Autodesk Inventor part; units mm, degrees
ref_plane "YZ Plane" through (0, 0, 0) normal (1, 0, 0) x (0, 1, 0)
ref_plane "XZ Plane" through (0, 0, 0) normal (0, 1, 0) x (-1, 0, 0)
ref_plane "XY Plane" through (0, 0, 0) normal (0, 0, 1) x (1, 0, 0)
sketch "Náčrt1" plane through (0, 0, 0) normal (0, 1, 0) x (-1, 0, 0)
  line L0 (0, -133.7) -> (0, 133.7)
  line L1 (-66.5, 0) -> (66.5, 0)
  line L2 (-47.5, 95.5) -> (47.5, 95.5)
  line L3 (47.5, 95.5) -> (47.5, -95.5)
  line L4 (47.5, -95.5) -> (-47.5, -95.5)
  line L5 (-47.5, -95.5) -> (-47.5, 95.5)
  line L6 (-47.5, 95.5) -> (47.5, -95.5) construction
  line L7 (47.5, 95.5) -> (-47.5, -95.5) construction
  point P0 (0, 0)
  dimension "d0" = 191
  dimension "d1" = 95
extrude "Vysunutí1" add sketch "Náčrt1" along normal blind 110
sketch "Náčrt2" plane through (0, 110, 0) normal (0, 1, 0) x (1, 0, 0)
  line L0 (0, 133.7) -> (0, -133.7)
  line L1 (66.5, 0) -> (-66.5, 0)
  circle A0 centre (0, -48) radius 42.5
  line L2 (-47.5, -95.5) -> (47.5, -95.5)
  point P0 (0, 0)
  dimension "d4" = 85
  dimension "d5" = 47.5
extrude "Vysunutí2" cut sketch "Náčrt2" against normal blind 85
sketch "Náčrt3" plane through (0, 110, 0) normal (0, 1, 0) x (1, 0, 0)
  line L0 (66.5, 0) -> (-66.5, 0)
  line L1 (0, 133.7) -> (0, -133.7)
  circle A0 centre (0, -48) radius 42.5
  line L2 (-42.5, -0.5) -> (42.5, -0.5)
  line L3 (42.5, -0.5) -> (42.5, 29.5)
  line L4 (42.5, 29.5) -> (-42.5, 29.5)
  line L5 (-42.5, 29.5) -> (-42.5, -0.5)
  point P0 (0, 0)
  dimension "d8" = 30
  dimension "d9" = 85
  dimension "d10" = 47.5
extrude "Vysunutí3" cut sketch "Náčrt3" against normal blind 105 contours L3 L2 L1 L0 | L0 L1 L4 L3 | L1 L2 L5 L0 | L0 L5 L4 L1
sketch "Náčrt4" plane through (0, 110, 0) normal (0, 1, 0) x (1, 0, 0)
  line L0 (0, 133.7) -> (0, -133.7)
  line L1 (66.5, 0) -> (-66.5, 0)
  line L2 (-42.5, 34.5) -> (42.5, 34.5)
  line L3 (42.5, 34.5) -> (42.5, 84.5)
  line L4 (42.5, 84.5) -> (-42.5, 84.5)
  line L5 (-42.5, 84.5) -> (-42.5, 34.5)
  line L6 (-42.5, 29.5) -> (42.5, 29.5)
  point P0 (0, 0)
  dimension "d13" = 5
  dimension "d14" = 50
  dimension "d15" = 85
extrude "Vysunutí4" cut sketch "Náčrt4" against normal blind 105
sketch "Náčrt6" plane through (0, 25, 48) normal (0, 1, 0) x (1, 0, 0)
  circle A0 centre (0, 0) radius 42.5
  line L0 (66.5, 48) -> (-66.5, 48)
  line L1 (0, 181.7) -> (0, -85.7)
  circle A1 centre (0, 0) radius 32.5
  point P0 (0, 48)
  dimension "d24" = 65
extrude "Vysunutí6" cut sketch "Náčrt6" against normal blind 10 contours A1 L1 | L1 A1
fillet "Zaoblení1" radius 8 4 edges at (47.5, 55, -95.5) (-47.5, 55, -95.5) (47.5, 55, 95.5) (-47.5, 55, 95.5)
fillet "Zaoblení2" radius 5 8 edges at (45.1569, 0, -93.1569) (0, 0, -95.5) (-45.1569, 0, -93.1569) (-47.5, 0, 0) (-45.1569, 0, 93.1569) (0, 0, 95.5) (45.1569, 0, 93.1569) (47.5, 0, 0)
sketch "Náčrt7" plane through (0, 110, 0) normal (0, 1, 0) x (1, 0, 0)
  line L0 (0, 133.7) -> (0, -133.7)
  line L1 (66.5, 0) -> (-66.5, 0)
  circle A0 centre (0, -48) radius 42.5
  line L2 (-45.5, -3.5) -> (45.5, -3.5)
  line L3 (45.5, -3.5) -> (45.5, 87.5)
  line L4 (45.5, 87.5) -> (-45.5, 87.5)
  line L5 (-45.5, 87.5) -> (-45.5, -3.5)
  point P0 (0, 0)
  dimension "d29" = 91
  dimension "d30" = 44.5
  dimension "d31" = 91
extrude "Vysunutí7" cut sketch "Náčrt7" against normal blind 3 contours L4 L3 L1 L0 | L0 L1 L5 L4 | L1 L3 L2 L0 | L0 L2 L5 L1
sketch "Náčrt8" plane through (42.5, 5, -34.5) normal (0, 0, -1) x (-1, 0, 0)
  line L0 (85, 102) -> (0, 102)
  line L1 (85, 102) -> (85, 0)
  circle A0 centre (73, 95) radius 3.5
  point P0 (42.5, -5)
  dimension "d34" = 7
  dimension "d35" = 12
  dimension "d36" = 3.5
extrude "Vysunutí8" cut sketch "Náčrt8" against normal blind 70
sketch "Náčrt9" plane through (42.5, 5, -34.5) normal (0, 0, -1) x (-1, 0, 0)
  line L0 (85, 102) -> (0, 102)
  line L1 (0, 102) -> (0, 0)
  line L2 (85, 102) -> (85, 0)
  point P0 (42.5, -5)
  point P1 (42.5, 92)
  dimension "d39" = 42.5
  dimension "d40" = 10
hole "Díra1" at (0, 97, -34.5) direction (0, 0, 1) diameter 3 depth 8 tip angle 118
sketch "Náčrt10" plane through (42.5, 5, 0.5) normal (0, 0, -1) x (-1, 0, 0)
  line L0 (85, 102) -> (0, 102)
  line L1 (0, 102) -> (0, 0)
  line L2 (85, 102) -> (85, 0)
  circle A0 centre (42.5, 92) radius 1.5
  point P0 (42.5, -5)
hole "Díra2" at (0, 97, 0.5) direction (0, 0, 1) diameter 3 depth 8 tip angle 118
properties part number "květináč"
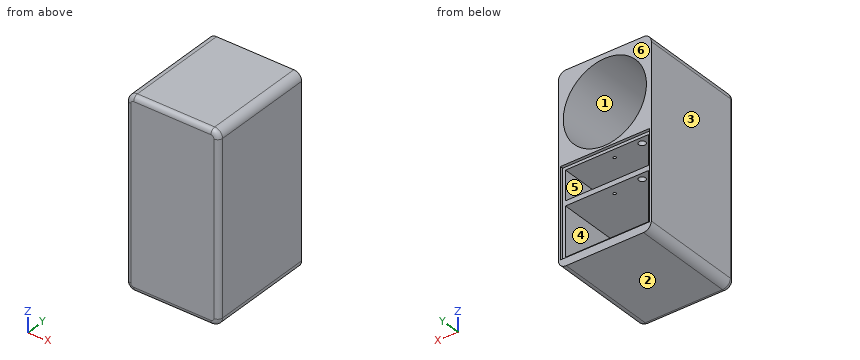
Can you work these out from the model? Positions are in its coordinate system, mm. Face numbers are marked on the shaded views. A direction names the side the tool comes from. Coordinates: 2 decimals unless noted, no trailing zeros. Write each loop counter-clockwise with the first axis right and the second up, starting at its lowest first coordinate (ties: lowest second). Pieces come first, ordered by that corner, then holes. Notation, with made-up numbers: M 67,43.25 L 79,43.25 A6 cw 79,47.25 Z; hole C -1.5,-7 d6. An arc over 180 degrees is marked long. Use one line per item in the form item = value.
Q1. If we section it at C-C (x = -30.5): State how many separate pieces and enclosed holes the cut face has, then the cut area to 3 significant figures.
Model answer:
separate_pieces = 3
enclosed_holes = 0
area = 7,150 mm^2
Q2. For P1, Ø1, axis at x = 1, z = -68.5, coming from the +Y side; P2, Ø19.5, axis at x = -14.5, z = 35.5, coming from the +Y side; P3, Ø5, axis at x = 4, z = -33.5, coming from the +Y side, each with a flat end and sliding along its axis, tell me the tip position at first contact or that it passes through.
Model answer:
P1 = 5
P2 = 15
P3 = 107
Q3. If we section it at A-A (y = 72.5): Write out the boundary of the cut face in (x, z), then the cut area to 3 significant figures.
Model answer:
outline = M -47.5,-87.5 A8 ccw -39.5,-95.5 L 39.5,-95.5 A8 ccw 47.5,-87.5 L 47.5,87.5 A8 ccw 39.5,95.5 L -39.5,95.5 A8 ccw -47.5,87.5 Z; hole M -42.5,-84.5 L 42.5,-84.5 L 42.5,-34.5 L -42.5,-34.5 Z; hole M -42.5,-29.5 L 42.5,-29.5 L 42.5,0.5 L -42.5,0.5 Z; hole C 0,48 d85
area = 5,620 mm^2
Q4. For the marked faces 1 and 2, which set-ups out of +Z, -Z, +X, -X, +Y, -Y let a thin tool reach every point of the face, with its end or its side?
Model answer:
face_1 = +Y
face_2 = -Z, +X, -X, +Y, -Y
Q5. We'd pull the mould along X, two halves only. Please class the marked faces 3, 4, 5 and 6: +X half, -X half, draft (parallel to the pull), parting line (faces both ways), or undercut.
Model answer:
face_3 = -X half
face_4 = undercut
face_5 = undercut
face_6 = draft
Q6. If we section it at D-D (z = 48): Write out the boundary of the cut face in (x, y).
Model answer:
outline = M -47.5,5 A5 ccw -42.5,0 L 42.5,0 A5 ccw 47.5,5 L 47.5,110 L 42.5,110 L 42.5,25 L 32.5,25 L 32.5,15 L -32.5,15 L -32.5,25 L -42.5,25 L -42.5,110 L -47.5,110 Z
Q7. If we section it at B-B (z = -15): Write out the boundary of the cut face in (x, y).
Model answer:
outline = M -47.5,5 A5 ccw -42.5,0 L 42.5,0 A5 ccw 47.5,5 L 47.5,110 L 45.5,110 L 45.5,107 L 42.5,107 L 42.5,5 L -42.5,5 L -42.5,107 L -45.5,107 L -45.5,110 L -47.5,110 Z
Q8. I need wall thicknesses on line 1 along Z through (x, y) = (-32, 13.5); line 2 along Y through (x, z) = (-30, 7); line 3 along X through (y, z) = (87, -7.5). Which ranges of each line are inside material? Lowest first, please. Write a range as from..to.
Model answer:
line_1 = -95.5..-84.5, -34.5..-29.5, 0.5..95.5
line_2 = 0..96.54, 103.46..110
line_3 = -47.5..-42.5, 42.5..47.5
